from build123d import *

# Parameters (mm, degrees)
SALIENTE_EXTRUIR1_DEPTH = 3
CORTAR_EXTRUIR1_REACH   = 5
CROQUIS2_W              = 10
CROQUIS2_H              = 18
CORTAR_EXTRUIR2_REACH   = 5
CROQUIS3_R              = 5
CROQUIS4_R              = 7
CROQUIS4_R_2            = 5
SALIENTE_EXTRUIR2_DEPTH = 40
CROQUIS5_R              = 7
SALIENTE_EXTRUIR3_DEPTH = 0.05
C_PULA1_FACE_RADIUS     = 7
C_PULA1_HEIGHT          = 6
REDONDEO1_R             = 2


with BuildPart() as part:
    # Croquis1 → Saliente-Extruir1 (new body)
    with BuildSketch(Plane(origin=(0, 155.4998128, 0), x_dir=(1, 0, 0), z_dir=(0, 1, 0))):
        with BuildLine():
            Line((1.881749032, 20.084971867), (1.881749032, 36.084971867))
            ThreePointArc((1.881749032, 36.084971867), (1.295962595, 37.499185429), (-0.118250968, 38.084971867))
            Line((-0.118250968, 38.084971867), (-5.118250968, 38.084971867))
            ThreePointArc((-5.118250968, 38.084971867), (-9.200733872, 40.198220521), (-9.832296176, 44.751638534))
            ThreePointArc((-9.832296176, 44.751638534), (-10.337546018, 48.394372944), (-13.603532342, 50.084971867))
            Line((-13.603532342, 50.084971867), (-45.118250968, 50.084971867))
            ThreePointArc((-45.118250968, 50.084971867), (-50.067998436, 48.034719335), (-52.118250968, 43.084971867))
            Line((-52.118250968, 43.084971867), (-52.118250968, 35.084971867))
            ThreePointArc((-52.118250968, 35.084971867), (-51.53246453, 33.670758305), (-50.118250968, 33.084971867))
            Line((-50.118250968, 33.084971867), (-48.118250968, 33.084971867))
            ThreePointArc((-48.118250968, 33.084971867), (-43.118250968, 28.084971867), (-48.118250968, 23.084971867))
            Line((-48.118250968, 23.084971867), (-50.118250968, 23.084971867))
            ThreePointArc((-50.118250968, 23.084971867), (-51.53246453, 22.499185429), (-52.118250968, 21.084971867))
            Line((-52.118250968, 21.084971867), (-52.118250968, 13.084971867))
            ThreePointArc((-52.118250968, 13.084971867), (-50.067998436, 8.135224399), (-45.118250968, 6.084971867))
            Line((-45.118250968, 6.084971867), (-13.603532342, 6.084971867))
            ThreePointArc((-13.603532342, 6.084971867), (-10.337546018, 7.77557079), (-9.832296176, 11.4183052))
            ThreePointArc((-9.832296176, 11.4183052), (-9.200733872, 15.971723213), (-5.118250968, 18.084971867))
            Line((-5.118250968, 18.084971867), (-0.118250968, 18.084971867))
            ThreePointArc((-0.118250968, 18.084971867), (1.295962595, 18.670758305), (1.881749032, 20.084971867))
        make_face()
    extrude(amount=SALIENTE_EXTRUIR1_DEPTH)

    # Croquis2 → Cortar-Extruir1 (cut, up to next)
    with BuildSketch(Plane(origin=(0, 158.4998128, 0), x_dir=(1, 0, 0), z_dir=(0, 1, 0)), mode=Mode.PRIVATE) as cortar_extruir1_sk1:
        with Locations((-22.118250968, 28.084971867)):
            Rectangle(CROQUIS2_W, CROQUIS2_H)
    cortar_extruir1_tool1 = extrude(cortar_extruir1_sk1.sketch, amount=-CORTAR_EXTRUIR1_REACH, mode=Mode.PRIVATE) & part.part
    add(cortar_extruir1_tool1.solids().sort_by_distance((-22.118251, 158.499813, -28.084972))[0], mode=Mode.SUBTRACT)

    # Croquis3 → Cortar-Extruir2 (cut, up to next)
    with BuildSketch(Plane(origin=(0, 158.4998128, 0), x_dir=(1, 0, 0), z_dir=(0, 1, 0)), mode=Mode.PRIVATE) as cortar_extruir2_sk1:
        with Locations((-35.318250968, 20.084971867)):
            Circle(CROQUIS3_R)
    cortar_extruir2_tool1 = extrude(cortar_extruir2_sk1.sketch, amount=-CORTAR_EXTRUIR2_REACH, mode=Mode.PRIVATE) & part.part
    add(cortar_extruir2_tool1.solids().sort_by_distance((-35.318251, 158.499813, -20.084972))[0], mode=Mode.SUBTRACT)

    # Croquis4 → Saliente-Extruir2 (add)
    with BuildSketch(Plane(origin=(0, 158.4998128, 0), x_dir=(1, 0, 0), z_dir=(0, 1, 0))):
        with Locations((-35.318250968, 20.084971867)):
            Circle(CROQUIS4_R)
        with Locations((-35.318250968, 20.084971867)):
            Circle(CROQUIS4_R_2, mode=Mode.SUBTRACT)
    extrude(amount=SALIENTE_EXTRUIR2_DEPTH)

    # Croquis5 → Saliente-Extruir3 (add)
    with BuildSketch(Plane(origin=(0, 198.4998128, 0), x_dir=(1, 0, 0), z_dir=(0, 1, 0))):
        with Locations((-35.318250968, 20.084971867)):
            Circle(CROQUIS5_R)
    extrude(amount=SALIENTE_EXTRUIR3_DEPTH)

    # Cúpula1: a dome of height H over a round flat face of radius A is a cap of a sphere of radius (A * A + H * H) / (2 * H)
    c_pula1_r = (C_PULA1_FACE_RADIUS * C_PULA1_FACE_RADIUS + C_PULA1_HEIGHT * C_PULA1_HEIGHT) / (2 * C_PULA1_HEIGHT)
    c_pula1_base = Plane((-35.318250968, 198.5498128, -20.084971867), z_dir=(0, 1, 0))
    with Locations(c_pula1_base.offset(C_PULA1_HEIGHT - c_pula1_r)):
        c_pula1_ball = Sphere(c_pula1_r, mode=Mode.PRIVATE)
    add(split(c_pula1_ball, bisect_by=c_pula1_base, keep=Keep.TOP, mode=Mode.PRIVATE))

    # Redondeo1
    redondeo1_edges = [part.edges().sort_by_distance(p)[0] for p in [
        (1.295962595, 158.4998128, -37.499185429),
        (-2.618250968, 158.4998128, -38.084971867),
        (-9.200733872, 158.4998128, -40.198220521),
        (-10.337546018, 158.4998128, -48.394372944),
        (-29.360891655, 158.4998128, -50.084971867),
        (-50.067998436, 158.4998128, -48.034719335),
        (-52.118250968, 158.4998128, -39.084971867),
        (-51.53246453, 158.4998128, -33.670758305),
        (-49.118250968, 158.4998128, -33.084971867),
        (-43.118250968, 158.4998128, -28.084971867),
        (1.295962595, 158.4998128, -18.670758305),
        (-49.118250968, 158.4998128, -23.084971867),
        (-51.53246453, 158.4998128, -22.499185429),
        (-52.118250968, 158.4998128, -17.084971867),
        (-50.067998436, 158.4998128, -8.135224399),
        (-29.360891655, 158.4998128, -6.084971867),
        (-10.337546018, 158.4998128, -7.77557079),
        (-9.200733872, 158.4998128, -15.971723213),
        (-2.618250968, 158.4998128, -18.084971867),
        (1.881749032, 158.4998128, -28.084971867),
    ]]
    fillet(redondeo1_edges, radius=REDONDEO1_R)


solid = part.part
Input: part model. Units: mm. Frame: model coordinates. A direction names the side the tool comes from. Give positions to 0.01 mm unless a question says otherwise; leave off trailing zeros. Order: outer loops, then holes, each group sorted by start corner. A loop starts at its lowest first (then second) coordinate and runs counter-clockwise, first axis right, second up. Notation, with made-up numbers: M -0.75,62 L 30.25,62 A34 cw 30.25,100 Z; hole C -36,15.25 d3. An arc over 180 degrees is marked long. Answer as a JSON object with one key per item and string values.
1. Cut plane A-A, the plane y = 182.5. Output: boundary loops of the cut face in (x, z).
Result sheet:
{"outline": "C -35.32,-20.08 d14; hole C -35.32,-20.08 d10"}
2. Cut plane B-B, the plane x = -31. Output: boundary loops of the cut face in (y, z), and give its area (3 significant figures).
Result sheet:
{"outline": "M 155.5,-50.08 L 156.5,-50.08 A2 ccw 158.5,-48.08 L 158.5,-25.59 L 198.55,-25.59 A5.61 ccw 198.55,-14.58 L 158.5,-14.58 L 158.5,-8.08 A2 ccw 156.5,-6.08 L 155.5,-6.08 L 155.5,-17.56 L 198.5,-17.56 L 198.5,-22.61 L 155.5,-22.61 Z", "area": "392 mm²"}
3. Reachability of faces 5 (the cylindrical face through (-49.104, 157.929, -33.686)), 6 (the cylindrical face through (-32.088, 178.244, -13.875)), 7 (the cylindrical face through (-2.653, 157.929, -37.484)) from +Z, -Z, +X, -X, +Y, -Y: full face, straight path, thin tool, end or side. Return the list, or none.
Result sheet:
{"face 5": "-X, +Y", "face 6": "+Y", "face 7": "-Z, +X, +Y"}
4. Pull-direction query (X, two-part tool) for faces 1 (the flat face through (-31, 155.5, -28)), 2 (the cylindrical face through (-10.307, 155.993, -48.35)), 3 (the flat face through (-35, 198.5, -20)), 4 (the flat face through (-27.118, 157, -28)); classes: +X half, -X half, draft (parallel to the pull), parting line (faces both ways), or undercut.
Result sheet:
{"face 1": "draft", "face 2": "+X half", "face 3": "undercut", "face 4": "undercut"}
5. Ray query, line 1 (Y direction, x = -22, z = -17); line 2 (X direction, y = 179, z = -16.5); line 3 (X direction, y = 176, z = -19.5). Return the intervals inside material, ascending. Write a range as [from, to].
Result sheet:
{"line 1": "[155.5, 158.5]", "line 2": "[-41.33, -38.8], [-31.83, -29.31]", "line 3": "[-42.29, -40.28], [-30.35, -28.34]"}
6. Cut plane C-C, the plane y = 201.5. Output: boundary loops of the cut face in (x, z), and give its area (3 significant figures).
Result sheet:
{"outline": "C -35.32,-20.08 d11.65", "area": "107 mm²"}
7. First-contact query: P1, Ø2, axis at x = -30, y = 177.5, coming from the -Z side; P2, Ø10, axis at y = 182, z = -31.5, coming from the +X side; P3, Ø20, axis at x = -27, z = -26.5, coming from the +Y side; P4, Ø1.5, axis at x = -27.5, y = 182.5, coming from the -Z side. Flat tips, straight axial feed; report the tip coordinate or a pass-through.
Result sheet:
{"P1": "z = -25.59", "P2": "x = -32.52", "P3": "y = 204.53", "P4": "through"}
